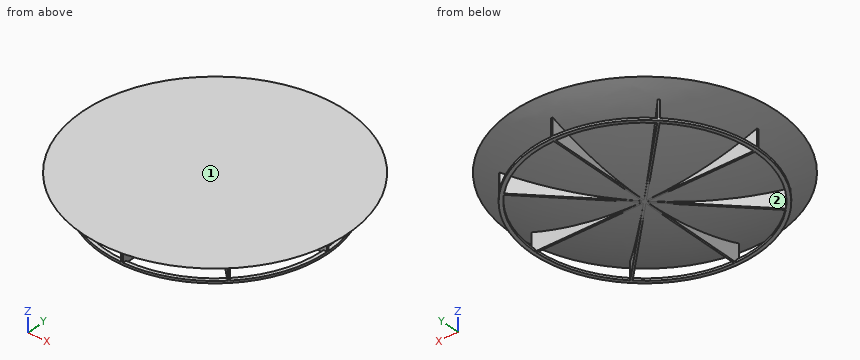
```python
from build123d import *

# Parameters (mm, degrees)
F0_W     = 25
F0_H     = 0.41
F1_DEPTH = 5
F3_COUNT = 8
F7_DEPTH = 0.5


with BuildPart() as f1:
    # F0 (on Top) → F1 (new body)
    with BuildSketch(Plane.XY):
        with Locations((-12.5, 0)):
            Rectangle(F0_W, F0_H)
    extrude(amount=F1_DEPTH)

    # F3: F1 ×8 about axis
    f3_axis = Axis((0, 0, 6.672881), (0, 0, 1))


with BuildPart() as f1_1:
    add(f1.part)
    for i in range(1, F3_COUNT):
        add(f1.part.rotate(f3_axis, i * 360 / F3_COUNT))

    # F4 (on Front) → F5 (revolve)
    with BuildSketch(Plane.XZ):
        with BuildLine():
            Line((0, 6), (-29.393877, 6))
            ThreePointArc((-29.393877, 6), (-15, 1.515308), (0, 0))
            Line((0, 0), (0, 6))
        make_face()
    revolve(axis=Axis((0, 0, 6.672881), (0, 0, 1)))

    # F6 (on Top) → F7 (join)
    with BuildSketch(Plane.XY):
        with BuildLine():
            ThreePointArc((-24.999159, -0.205), (0.102501, -24.99979), (25, 0))
            ThreePointArc((25, 0), (0.102501, 24.99979), (-24.999159, 0.205))
            Line((-24.999159, 0.205), (-24.199132, 0.205))
            ThreePointArc((-24.199132, 0.205), (0.102501, 24.199783), (24.2, 0))
            ThreePointArc((24.2, 0), (0.102501, -24.199783), (-24.199132, -0.205))
            Line((-24.199132, -0.205), (-24.999159, -0.205))
        make_face()
        with BuildLine():
            ThreePointArc((-25, 0), (-24.99979, 0.102501), (-24.999159, 0.205))
            Line((-24.999159, 0.205), (-25, 0.205))
            Line((-25, 0.205), (-25, 0))
        make_face()
        with BuildLine():
            Line((-25, -0.205), (-24.999159, -0.205))
            ThreePointArc((-24.999159, -0.205), (-24.99979, -0.102501), (-25, 0))
            Line((-25, 0), (-25, -0.205))
        make_face()
    extrude(amount=F7_DEPTH)


solid = f1_1.part
```
Input: part model. Units: mm. Frame: model coordinates. Face numbers are marked on the shaded views. Give positions to 0.01 mm unless a question says otherwise; leave off trailing zeros. Return JSON: item names as keys, results as strings.
1) Section query A-A on y = -19.5. Count the separate pieces of the cut face and the enclosed holes in it, and give its area (3 significant figures).
Taken from the geometry:
{"separate pieces": "3", "enclosed holes": "0", "area": "103 mm2"}
2) Line query: L1, parallel to Y at x = 23, z = 2 (3 decimals); L2, parallel to Z at x = -24.5, y = 4.5. Output: solid intervals per line, ascending. Write a range as [from, to].
Taken from the geometry:
{"L1": "y = [-0.205, 0.205]", "L2": "z = [0, 0.5], [4.26, 6]"}
3) Mould query, pull axis Y, two halves, no side actions, for the marked faces 1 and 2. Classes: released by +Y, released by -Y, zero draft, split by the parting line, or undercut.
Taken from the geometry:
{"face 1": "zero draft", "face 2": "undercut"}
4) Contact query for flat-ended pins moving along their axis: pin 1 (1 mm diameter, centred on x = -18, y = 19, fed in from -Z); pin 2 (3.5 mm diameter, centred on y = 14, z = 1.5, fed in from +X); pin 3 (2 mm diameter, centred on y = -11.5, z = 1, fed in from +X). Output: stop coordinate, or through.
Taken from the geometry:
{"pin 1": "stops at z = 4.53", "pin 2": "stops at x = 21.61", "pin 3": "stops at x = 22.63"}
